```python
from build123d import *

# Parameters (mm, degrees)
BOSS_EXTRUDE1_START     = -73.056856187
BOSS_EXTRUDE1_OUTLINE_W = 38.1
BOSS_EXTRUDE1_OUTLINE_H = 76.2
BOSS_EXTRUDE1_DEPTH     = 152.4
SKETCH3_W               = 34.29
SKETCH3_H               = 25.4
CUT_EXTRUDE1_DEPTH      = 116.642749409
SKETCH4_W               = 17.78
SKETCH4_H               = 6.35
CUT_EXTRUDE2_DEPTH      = 116.642749409
CUT_EXTRUDE3_DEPTH      = 116.642749409
CUT_EXTRUDE4_DEPTH      = 116.642749409
CUT_EXTRUDE5_DEPTH      = 116.642749409
CUT_EXTRUDE5_DEPTH_BACK = 116.642749409
SKETCH8_R               = 6.35
CUT_EXTRUDE6_DEPTH      = 117.419003905
CUT_EXTRUDE6_DEPTH_BACK = 117.419003905
SKETCH11_R              = 8.255
CUT_EXTRUDE7_DEPTH      = 116.579441005
CUT_EXTRUDE7_DEPTH_BACK = 116.579441005
CUT_EXTRUDE9_DEPTH      = 116.579441005
CUT_EXTRUDE9_DEPTH_BACK = 116.579441005
SKETCH14_W              = 3.443454538
SKETCH14_H              = 25.4


# Read off the part's stored shape, not the designer's step: Boss-Extrude1
with BuildPart() as part:
    # Boss-Extrude1 outline → Boss-Extrude1 (new body)
    with BuildSketch(Plane.YZ.offset(BOSS_EXTRUDE1_START)):
        with Locations((-16.607692308, 38.1)):
            Rectangle(BOSS_EXTRUDE1_OUTLINE_W, BOSS_EXTRUDE1_OUTLINE_H)
    extrude(amount=BOSS_EXTRUDE1_DEPTH)

    # Sketch3 → Cut-Extrude1 (cut, through all)
    with BuildSketch(Plane.XY.offset(76.2)):
        with Locations((-55.911856187, -22.957692308)):
            Rectangle(SKETCH3_W, SKETCH3_H)
    extrude(amount=-CUT_EXTRUDE1_DEPTH, mode=Mode.SUBTRACT)

    # Sketch4 → Cut-Extrude2 (cut, through all)
    with BuildSketch(Plane.XY.offset(76.2)):
        with Locations((-29.876856187, -32.482692308)):
            Rectangle(SKETCH4_W, SKETCH4_H)
    extrude(amount=-CUT_EXTRUDE2_DEPTH, mode=Mode.SUBTRACT)

    # Sketch5 → Cut-Extrude3 (cut, through all)
    with BuildSketch(Plane.XY.offset(76.2)):
        Polygon((-20.986856187, -35.657692308), (-20.986856187, -10.257692308), (79.343143813, -35.657692308), align=None)
    extrude(amount=-CUT_EXTRUDE3_DEPTH, mode=Mode.SUBTRACT)

    # Sketch6 → Cut-Extrude4 (cut, through all)
    with BuildSketch(Plane.XY.offset(76.2)):
        Polygon((79.343143813, 2.442307692), (79.343143813, -22.957692308), (-10.826856187, 2.442307692), align=None)
    extrude(amount=-CUT_EXTRUDE4_DEPTH, mode=Mode.SUBTRACT)

    # Sketch8 → Cut-Extrude5 (cut, two sides: drawn at the far end of the back side and taken through both)
    with BuildSketch(Plane(origin=(0, 0, 0), x_dir=(1, 0, 0), z_dir=(0, 1, 0)).offset(-CUT_EXTRUDE5_DEPTH_BACK)):
        with Locations(Location((-54.006856187, -57.15, 0), (0, 0, 270))):
            Circle(SKETCH8_R)
    extrude(amount=CUT_EXTRUDE5_DEPTH + CUT_EXTRUDE5_DEPTH_BACK, mode=Mode.SUBTRACT)

    # Sketch11 → Cut-Extrude6 (cut, two sides: drawn at the far end of the back side and taken through both)
    with BuildSketch(Plane(origin=(0, 2.442307692, 0), x_dir=(1, 0, 0), z_dir=(0, 1, 0)).offset(-CUT_EXTRUDE6_DEPTH_BACK)):
        with Locations(Location((-54.006856187, -19.05, 0), (0, 0, 270))):
            Circle(SKETCH11_R)
    extrude(amount=CUT_EXTRUDE6_DEPTH + CUT_EXTRUDE6_DEPTH_BACK, mode=Mode.SUBTRACT)

    # Sketch12 → Cut-Extrude7 (cut, two sides: drawn at the far end of the back side and taken through both)
    with BuildSketch(Plane(origin=(-0.158549081, -0.562849239, 0), x_dir=(0.9625404418449637, -0.2711381526323841, 0), z_dir=(0.27113815263238417, 0.9625404418449638, 0)).offset(-CUT_EXTRUDE7_DEPTH_BACK)):
        with BuildLine():
            ThreePointArc((14.316510266, -19.05), (7.966510266, -25.4), (1.616510266, -19.05))
            Line((1.616510266, -19.05), (1.616510266, -57.15))
            ThreePointArc((1.616510266, -57.15), (7.966510266, -50.8), (14.316510266, -57.15))
            Line((14.316510266, -57.15), (14.316510266, -19.05))
        make_face()
        with BuildLine():
            ThreePointArc((14.316510266, -19.05), (7.966510266, -12.7), (1.616510266, -19.05))
            Line((1.616510266, -19.05), (14.316510266, -19.05))
        make_face()
        with BuildLine():
            Line((14.316510266, -19.05), (1.616510266, -19.05))
            ThreePointArc((1.616510266, -19.05), (7.966510266, -25.4), (14.316510266, -19.05))
        make_face()
        with BuildLine():
            ThreePointArc((14.316510266, -57.15), (7.966510266, -50.8), (1.616510266, -57.15))
            Line((1.616510266, -57.15), (14.316510266, -57.15))
        make_face()
        with BuildLine():
            Line((14.316510266, -57.15), (1.616510266, -57.15))
            ThreePointArc((1.616510266, -57.15), (7.966510266, -63.5), (14.316510266, -57.15))
        make_face()
    extrude(amount=CUT_EXTRUDE7_DEPTH + CUT_EXTRUDE7_DEPTH_BACK, mode=Mode.SUBTRACT)

    # Sketch14 → Cut-Extrude9 (cut, two sides: drawn at the far end of the back side and taken through both)
    with BuildSketch(Plane(origin=(-0.158549081, -0.562849239, 0), x_dir=(0.9625404418449637, -0.2711381526323841, 0), z_dir=(0.27113815263238417, 0.9625404418449638, 0)).offset(-CUT_EXTRUDE9_DEPTH_BACK)):
        with Locations((84.317418253, -38.1)):
            Rectangle(SKETCH14_W, SKETCH14_H)
        with BuildLine():
            Line((82.595690984, -25.4), (33.366510266, -25.4))
            ThreePointArc((33.366510266, -25.4), (42.346766387, -29.119743879), (46.066510266, -38.1))
            ThreePointArc((46.066510266, -38.1), (42.346766387, -47.080256121), (33.366510266, -50.8))
            Line((33.366510266, -50.8), (82.595690984, -50.8))
            Line((82.595690984, -50.8), (82.595690984, -25.4))
        make_face()
        with BuildLine():
            ThreePointArc((46.066510266, -38.1), (42.346766387, -29.119743879), (33.366510266, -25.4))
            Line((33.366510266, -25.4), (33.366510266, -50.8))
            ThreePointArc((33.366510266, -50.8), (42.346766387, -47.080256121), (46.066510266, -38.1))
        make_face()
        with BuildLine():
            Line((33.366510266, -50.8), (33.366510266, -25.4))
            ThreePointArc((33.366510266, -25.4), (20.666510266, -38.1), (33.366510266, -50.8))
        make_face()
    extrude(amount=CUT_EXTRUDE9_DEPTH + CUT_EXTRUDE9_DEPTH_BACK, mode=Mode.SUBTRACT)


solid = part.part
```
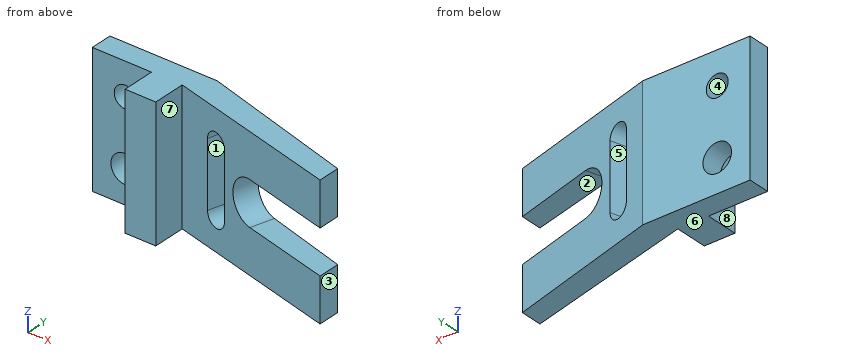
Can you work these out from the model? Positions are in its coordinate system, mm. Face numbers are marked on the shaded views. A direction names the side the tool comes from. Coordinates: 2 decimals unless noted, no trailing zeros. Loops run counter-clockwise (first coordinate to the right, second up) from the corner with the lowest first, then second, coordinate; pieces in that order, holes last. Notation, with made-up numbers: (-27, 89) - (-12, 89) arc R6 cw to (-12, 95) - close; hole circle Ø8 at (16.25, 17). An arc over 180 degrees is marked (long way). Answer as CSV lines item,"result". Start each with the question number.
1) Suppose I cut it at D-D (x = -29.5). Please give me the cut outline in (y, z).
2) For pin 1 (10 mm diameter, centred on x = 15, z = 64, fed in from +Y); pin 2 (19.5 mm diameter, centred on x = -32, z = 26.5, fed in from -Y); pin 3 (9.5 mm diameter, centred on y = -21, z = 38.5, fed in from -X), each with a flat end and sliding along its axis, tell me the tip position at first contact or that it passes through.
3) Thinking about a two-plate mould opening in X: for the marked faces 1, 2 and 3, which applies, pulls with the +X half, pulls with the -X half, needs draft (parallel to the pull), parting line crosses it, or undercut?
4) Which directions (+Z, -Z, +X, -X, +Y, -Y) give clear straight access to the entire face, cutting with the end or side of a thin tool? Please do the marked faces 4, 5, 6, 7 and 8.
5) Suppose I cut it at C-C (y = -27). Please give me the cut outline in (x, z), plus the area to 3 significant figures.
6) Suppose I cut it at B-B (x = 63). Please give me the cut outline in (y, z), plus the area to 3 significant figures.
7) Suppose I cut it at A-A (z = 67.5). Please give me the cut outline in (x, y), plus the area to 3 significant figures.
8) I need wall thicknesses on line 1 (Z direction, x = 62.5, y = -25); line 2 (Y direction, x = -61.5, z = 69); line 3 (Z direction, x = -52.5, y = -7). Which ranges of each line are inside material? Lowest first, please. Write a range as from..to.
Check result:
1,outline,"(-29.31, 0) - (2.44, 0) - (2.44, 76.2) - (-29.31, 76.2) - close"
2,pin 1,"stops at y = -3.42"
2,pin 2,"stops at y = -29.31"
2,pin 3,"stops at x = -38.77"
3,face 1,"undercut"
3,face 2,"needs draft"
3,face 3,"pulls with the +X half"
4,face 4,"+Y, -Y"
4,face 5,"+Y"
4,face 6,"-Z, +X, -X, +Y, -Y"
4,face 7,"+Z, -Z, -Y"
4,face 8,"+Z, -Z, -X, -Y"
5,outline,"(-38.77, 0) - (-20.99, 0) - (-20.99, 76.2) - (-38.77, 76.2) - close; (45.15, 0) - (79.34, 0) - (79.34, 25.4) - (45.15, 25.4) - close; (45.15, 50.8) - (79.34, 50.8) - (79.34, 76.2) - (45.15, 76.2) - close"
5,area,"3,090 mm²"
6,outline,"(-31.52, 0) - (-18.35, 0) - (-18.35, 25.4) - (-31.52, 25.4) - close; (-31.52, 50.8) - (-18.35, 50.8) - (-18.35, 76.2) - (-31.52, 76.2) - close"
6,area,"669 mm²"
7,outline,"(-73.06, -10.26) - (-38.77, -10.26) - (-38.77, -29.31) - (-20.99, -29.31) - (-20.99, -10.26) - (79.34, -35.66) - (79.34, -22.96) - (-10.83, 2.44) - (-73.06, 2.44) - close"
7,area,"2,400 mm²"
8,line 1,"z = 0..25.4, 50.8..76.2"
8,line 2,"y = -10.26..2.44"
8,line 3,"z = 0..10.93, 27.17..50.98, 63.32..76.2"
